The listing builds one solid part. Answer for the finished solid, in the listing's coordinates (mm). A direction names the side the tool comes from. Give positions to 0.01 mm unless a question says otherwise; leave off trailing zeros. Order: outer loops, then holes, each group sorted by start corner. A loop starts at its lowest first (then second) coordinate and runs counter-clockwise, first axis right, second up. Notation, with made-up numbers: (74, 66.5) - (83, 66.5) arc R26 ccw to (83, 105.5) - close; hole circle Ø1 at (56, 11). An arc over 180 degrees is marked (long way). Write each question's results on one line, items separated by ' | '. Start each with the question number.
1. Section B-B (z = -12.5) is taken. Give the vertices of the cut face in (x, y).
2. Find the intervals of material crossed by L1, parallel to X at y = 3.25, z = -12.5; L2, parallel to Z at x = 23.5, y = 4.5; L3, parallel to X at y = 8, z = -12.5, in increasing order.
3. Determine the mould class of faces 1 (the face through (19, 0, -13)), 2 (the face through (28, 4, 0)), 3 (the face through (20.6, 5.6, -12.6)) for opening direction Z: released by +Z, released by -Z, zero draft, split by the parting line, or undercut.
4. Flat-ended cylindrical pins translate along their axes: pin 1 (5.5 mm diameter, centred on x = 32.5, z = -16.5, fed in from +Y); pin 2 (13 mm diameter, centred on x = 7.5, z = -8.5, fed in from +Y); pin 3 (1.8 mm diameter, centred on y = 8.5, z = -10, fed in from -X). Find the tip coordinate at first contact, or state that the pin passes through.
5. Section C-C (y = 8.25) is taken. Give the vertices of the cut face in (x, z), and give its area (3 significant figures).
6. Section A-A (x = 23.5) is taken. Give the vertices of the cut face in (y, z), and give its area (3 significant figures).
7. Which of the six approach directions +Z, -Z, +X, -X, +Y, -Y give full straight-line access (tool end or side, diameter ignored) to faces 4 (the face through (18.785, 7.958, -24.699)), 5 (the face through (27.699, 10.014, -24.715)), 6 (the face through (18.785, 8.042, -0.301)), 7 (the face through (18.5, 8, -12)), 8 (the face through (28, 10, -12))?
8. Section D-D (z = -22.25) is taken. Give the vertices of the cut face in (x, y), and give its area (3 significant figures).
from build123d import *

# Parameters (mm, degrees)
SKETCH1_W            = 45
SKETCH1_H            = 25
BOSS_EXTRUDE1_DEPTH  = 5
SKETCH5_W            = 26.5
SKETCH5_H            = 25
BOSS_EXTRUDE3_DEPTH  = 4
SKETCH11_W           = 9.5
SKETCH11_H           = 25
BOSS_EXTRUDE5_DEPTH  = 2
SKETCH12_W           = 3
SKETCH12_H           = 25
CUT_EXTRUDE2_DEPTH   = 52.826634079
M5_CLEARANCE_HOLE1_D = 5.8
FILLET2_R            = 1


with BuildPart() as part:
    # Sketch1 → Boss-Extrude1 (new body)
    with BuildSketch(Plane(origin=(0, 0, 0), x_dir=(1, 0, 0), z_dir=(0, 1, 0))):
        with Locations((22.5, 12.5)):
            Rectangle(SKETCH1_W, SKETCH1_H)
    extrude(amount=BOSS_EXTRUDE1_DEPTH)

    # Sketch5 → Boss-Extrude3 (add)
    with BuildSketch(Plane(origin=(0, 5, 0), x_dir=(1, 0, 0), z_dir=(0, 1, 0))):
        with Locations((31.75, 12.5)):
            Rectangle(SKETCH5_W, SKETCH5_H)
    extrude(amount=BOSS_EXTRUDE3_DEPTH)

    # Sketch11 → Boss-Extrude5 (add)
    with BuildSketch(Plane(origin=(0, 9, 0), x_dir=(1, 0, 0), z_dir=(0, 1, 0))):
        with Locations((23.25, 12.5)):
            Rectangle(SKETCH11_W, SKETCH11_H)
    extrude(amount=BOSS_EXTRUDE5_DEPTH)

    # Sketch12 → Cut-Extrude2 (cut, through all)
    with BuildSketch(Plane(origin=(0, 5, 0), x_dir=(1, 0, 0), z_dir=(0, 1, 0))):
        with Locations((1.5, 12.5)):
            Rectangle(SKETCH12_W, SKETCH12_H)
    extrude(amount=-CUT_EXTRUDE2_DEPTH, mode=Mode.SUBTRACT)

    # M5 Clearance Hole1 (through all)
    with Locations(Plane(origin=(0, 0, 0), x_dir=(-1, 0, 0), z_dir=(0, -1, 0))):
        with Locations((-23.5, 12.5)):
            Hole(M5_CLEARANCE_HOLE1_D / 2)

    # Fillet2
    fillet2_edges = [part.edges().sort_by_distance(p)[0] for p in [
        (18.5, 8, -25),
        (18.5, 8, 0),
        (28, 10, 0),
        (28, 10, -25),
        (3, 2.5, -25),
        (3, 2.5, 0),
        (45, 4.5, -25),
        (45, 4.5, 0),
    ]]
    fillet(fillet2_edges, radius=FILLET2_R)


solid = part.part
Reported:
1) outline: (3, 0) - (20.6, 0) - (20.6, 11) - (18.5, 11) - (18.5, 5) - (3, 5) - close; (26.4, 0) - (45, 0) - (45, 9) - (28, 9) - (28, 11) - (26.4, 11) - close
2) L1: 3 to 20.6, 26.4 to 45 | L2: -25 to -15.4, -9.6 to 0 | L3: 18.5 to 20.6, 26.4 to 45
3) face 1: zero draft | face 2: released by +Z | face 3: undercut
4) pin 1: y = 9 | pin 2: y = 5 | pin 3: x = 18.5
5) outline: (18.5, -24) arc R1 ccw to (19.5, -25) - (44, -25) arc R1 ccw to (45, -24) - (45, -1) arc R1 ccw to (44, 0) - (19.5, 0) arc R1 ccw to (18.5, -1) - close; hole circle Ø5.8 at (23.5, -12.5) | area: 635 mm²
6) outline: (0, -25) - (11, -25) - (11, -15.4) - (0, -15.4) - close; (0, -9.6) - (11, -9.6) - (11, 0) - (0, 0) - close | area: 211 mm²
7) face 4: -Z, -X, +Y | face 5: -Z, +X, +Y | face 6: +Z, -X, +Y | face 7: +Z, -Z, -X, +Y | face 8: +Z, -Z, +X, +Y
8) outline: (3, 0) - (45, 0) - (45, 9) - (28, 9) - (28, 11) - (18.5, 11) - (18.5, 5) - (3, 5) - close | area: 335 mm²
